Autodesk Inventor part; units mm, degrees
ref_plane "YZ Plane" through (0, 0, 0) normal (1, 0, 0) x (0, 1, 0)
ref_plane "XZ Plane" through (0, 0, 0) normal (0, 1, 0) x (-1, 0, 0)
ref_plane "XY Plane" through (0, 0, 0) normal (0, 0, 1) x (1, 0, 0)
sketch "Esboço1" plane through (0, 0, 0) normal (0, 1, 0) x (-1, 0, 0)
  line L0 (0, 0) -> (22, 0)
  line L1 (22, 0) -> (22, -23.4641)
  line L2 (22, -24) -> (25.6764, -24) construction
  line L3 (0, 0) -> (0, -23.4641)
  line L4 (1.9, -27.8268) -> (1.9, -102.1732)
  line L5 (0, -106.5359) -> (0, -130)
  line L6 (0, -130) -> (22, -130)
  line L7 (22, -130) -> (22, -106.5359)
  line L8 (20.1, -102.1732) -> (20.1, -27.8268)
  line L9 (21.7321, -24.4641) -> (20.3679, -26.8268)
  line L10 (1.6321, -26.8268) -> (0.2679, -24.4641)
  line L11 (20.3679, -103.1732) -> (21.7321, -105.5359)
  line L12 (0.2679, -105.5359) -> (1.6321, -103.1732)
  arc A0 (21.7321, -24.4641) -> (22, -23.4641) centre (20, -23.4641) ccw
  arc A1 (20.3679, -26.8268) -> (20.1, -27.8268) centre (22.1, -27.8268) ccw
  arc A2 (1.9, -27.8268) -> (1.6321, -26.8268) centre (-0.1, -27.8268) ccw
  arc A3 (0, -23.4641) -> (0.2679, -24.4641) centre (2, -23.4641) ccw
  arc A4 (22, -106.5359) -> (21.7321, -105.5359) centre (20, -106.5359) ccw
  arc A5 (20.1, -102.1732) -> (20.3679, -103.1732) centre (22.1, -102.1732) ccw
  arc A6 (1.6321, -103.1732) -> (1.9, -102.1732) centre (-0.1, -102.1732) ccw
  arc A7 (0.2679, -105.5359) -> (0, -106.5359) centre (2, -106.5359) ccw
  line L13 (7.5, -52.4035) -> (7.5, -77.5965)
  spline S0 degree 3 poles (7.5, -52.4035) (7.1712, -52.2005) (6.8736, -51.9509) (6.3593, -51.374) (6.1453, -51.0498) (5.8168, -50.3503) (5.704, -49.9786) (5.5886, -49.2144) (5.5866, -48.826) (5.6404, -48.4433) knots -0.463747 -0.463747 -0.463747 -0.463747 -0.347807 -0.347807 -0.231874 -0.231874 -0.115941 -0.115941 -0.000001 -0.000001 -0.000001 -0.000001
  line L14 (5.6404, -48.4433) -> (6.2661, -43.9914)
  spline S1 degree 3 poles (6.2661, -43.9914) (6.3326, -43.5177) (6.4837, -43.0598) (6.9401, -42.2191) (7.2419, -41.8431) (7.9639, -41.2155) (8.3783, -40.9689) (9.2743, -40.6339) (9.7488, -40.5481) (10.2271, -40.5481) knots -0.574004 -0.574004 -0.574004 -0.574004 -0.430503 -0.430503 -0.287003 -0.287003 -0.143502 -0.143502 -0.000001 -0.000001 -0.000001 -0.000001
  line L15 (10.2271, -40.5481) -> (11.7729, -40.5481)
  spline S2 degree 3 poles (11.7729, -40.5481) (12.2512, -40.5481) (12.7257, -40.6339) (13.6217, -40.9689) (14.0361, -41.2155) (14.7581, -41.8431) (15.0599, -42.2191) (15.5163, -43.0598) (15.6674, -43.5177) (15.7339, -43.9914) knots -0.574004 -0.574004 -0.574004 -0.574004 -0.430503 -0.430503 -0.287003 -0.287003 -0.143502 -0.143502 -0.000001 -0.000001 -0.000001 -0.000001
  line L16 (15.7339, -43.9914) -> (16.3596, -48.4433)
  spline S3 degree 3 poles (16.3596, -48.4433) (16.4134, -48.826) (16.4114, -49.2144) (16.296, -49.9786) (16.1832, -50.3503) (15.8547, -51.0498) (15.6407, -51.374) (15.1264, -51.9509) (14.8288, -52.2005) (14.5, -52.4035) knots -0.463747 -0.463747 -0.463747 -0.463747 -0.347807 -0.347807 -0.231874 -0.231874 -0.115941 -0.115941 -0.000001 -0.000001 -0.000001 -0.000001
  line L17 (14.5, -77.5965) -> (14.5, -52.4035)
  spline S4 degree 3 poles (14.5, -77.5965) (14.8288, -77.7995) (15.1264, -78.0491) (15.6407, -78.626) (15.8547, -78.9502) (16.1832, -79.6497) (16.296, -80.0214) (16.4114, -80.7856) (16.4134, -81.174) (16.3596, -81.5567) knots -0.463747 -0.463747 -0.463747 -0.463747 -0.347807 -0.347807 -0.231874 -0.231874 -0.115941 -0.115941 -0.000001 -0.000001 -0.000001 -0.000001
  line L18 (15.7339, -86.0086) -> (16.3596, -81.5567)
  spline S5 degree 3 poles (15.7339, -86.0086) (15.6674, -86.4823) (15.5163, -86.9402) (15.0599, -87.7809) (14.7581, -88.1569) (14.0361, -88.7845) (13.6217, -89.0311) (12.7257, -89.3661) (12.2512, -89.4519) (11.7729, -89.4519) knots -0.574004 -0.574004 -0.574004 -0.574004 -0.430503 -0.430503 -0.287003 -0.287003 -0.143502 -0.143502 -0.000001 -0.000001 -0.000001 -0.000001
  spline S6 degree 3 poles (10.2271, -89.4519) (9.7488, -89.4519) (9.2743, -89.3661) (8.3783, -89.0311) (7.9639, -88.7845) (7.2419, -88.1569) (6.9401, -87.7809) (6.4837, -86.9402) (6.3326, -86.4823) (6.2661, -86.0086) knots -0.574004 -0.574004 -0.574004 -0.574004 -0.430503 -0.430503 -0.287003 -0.287003 -0.143502 -0.143502 -0.000001 -0.000001 -0.000001 -0.000001
  line L19 (10.2271, -89.4519) -> (11.7729, -89.4519)
  line L20 (5.6404, -81.5567) -> (6.2661, -86.0086)
  spline S7 degree 3 poles (5.6404, -81.5567) (5.5866, -81.174) (5.5886, -80.7856) (5.704, -80.0214) (5.8168, -79.6497) (6.1453, -78.9502) (6.3593, -78.626) (6.8736, -78.0491) (7.1712, -77.7995) (7.5, -77.5965) knots -0.463747 -0.463747 -0.463747 -0.463747 -0.347807 -0.347807 -0.231874 -0.231874 -0.115941 -0.115941 -0.000001 -0.000001 -0.000001 -0.000001
  point P0 (20.1, -27.2909)
  point P1 (0, -24)
  point P2 (1.9, -27.2909)
  point P3 (0, -106)
  point P4 (22, -106)
  point P5 (20.1, -102.7091)
  point P6 (11, -130)
  point P7 (11, -89.4519)
  point P8 (11, -40.5481)
  point P9 (20.1, -65)
  point P10 (14.5, -65)
  dimension "d0" = 22
  dimension "d1" = 24
  dimension "d4" = 3.8
  dimension "d6" = 3.8
  dimension "d7" = 24
  dimension "d8" = 18.2
  dimension "d10" = 0
  dimension "d11" = 130
  dimension "d12" = 1.9
  dimension "d13" = 2
  dimension "d14" = 2
  dimension "d38" = 7
  dimension "d39" = 7
  dimension "d40" = 4.4957
  dimension "d41" = 4.4957
  dimension "d42" = 4.4519
  dimension "d43" = 0.6257
  dimension "d44" = 172
  dimension "d45" = 1.5457
  dimension "d46" = 1.5457
  dimension "d47" = 0.6257
  dimension "d48" = 4.4519
  dimension "d49" = 3.9611
  dimension "d50" = 3.4433
  dimension "d51" = 9.4679
  dimension "d52" = 3.9611
  dimension "d53" = 3.9602
  dimension "d54" = 1.8596
  dimension "d55" = 4.4519
  dimension "d56" = 3.9602
  dimension "d57" = 3.9602
  dimension "d58" = 4.3751
  dimension "d59" = 1.8596
  dimension "d60" = 3.9611
  dimension "d61" = 3.9611
  dimension "d62" = 3.4433
  dimension "d63" = 3.4433
  dimension "d64" = 0
  dimension "d65" = 48.9038
  dimension "d67" = 0
extrude "Extrusão1" add sketch "Esboço1" along normal blind 25.4
sketch "Esboço2" plane through (0, 0, 0) normal (1, 0, 0) x (0, 0, -1)
  line L0 (0, 0) -> (0, 25.4)
  line L1 (0, 25.4) -> (23.4641, 25.4)
  line L2 (130, 0) -> (130, 25.4)
  line L3 (106.5359, 25.4) -> (130, 25.4)
  point P0 (12, 20.2)
  point P1 (12, 5.2)
  point P2 (118, 20.2)
  point P3 (118, 5.2)
  point P4 (11.7321, 25.4)
  dimension "d70" = 15
  dimension "d72" = 25.4
  dimension "d73" = 5.2
  dimension "d74" = 0
  dimension "d75" = 12
  dimension "d76" = 15
  dimension "d77" = 12
  dimension "d78" = 0
  dimension "d79" = 5.2
hole "Furo1" at (0, 20.2, -12) at (0, 5.2, -12) at (0, 20.2, -118) at (0, 5.2, -118) direction (-1, 0, 0) diameter 5 end through all
equation "\"d85\" = Espessura"
equation "\"Raio_vergadura\" = Espessura"
equation "\"Largura_alívio_de_vergadura\" = Espessura"
equation "\"Profundidade_alívio_de_vergadura\" = 0.5 * Espessura"
equation "\"Tamanho_alívio_de_dobra\" = 4 * Espessura"
equation "\"Remanescente_mínimo\" = 2 * Espessura"
equation "\"Raiodetransição\" = Raio_vergadura"
equation "\"Tamanho_de_raio_de_Jacobi\" = Raio_vergadura"
equation "\"TamanhoFolga\" = Espessura"
properties part number "Célula de carga" material "Alumínio 6061"
Could you check a few things on this model? Use its own coordinates, in mm. A direction names the side the tool comes from. Round coordinates to 2 decimals unless told otherwise and drop trailing zeros. Loops run counter-clockwise (first coordinate to the right, second up) from the corner with the lowest first, then second, coordinate; pieces in that order, holes last. Notation, with made-up numbers: (54.5, -20.75) -> (107.5, -20.75) arc R32 ccw to (107.5, 16.25) -> close; hole circle Ø2 at (46.5, 87.25). An arc over 180 degrees is marked (long way). One line per question, with ' | ' between items.
(1) For pin 1 Ø8 at (x, z) = (-8.5, -73) entering from -Y; pin 2 Ø3 at (y, z) = (20.5, -86) entering from +X; pin 3 Ø12 at (y, z) = (10.5, -81) entering from -X, each with a flat end and sliding along its axis, tell me the tip position at first contact or that it passes through.
Model answer:
pin 1: stops at y = 0 | pin 2: stops at x = -1.9 | pin 3: stops at x = -20.1
(2) If we section it at D-D on x = -18.75: List the corners of the cut face in (y, z) for me.
Model answer:
outline: (0, -130) -> (25.4, -130) -> (25.4, 0) -> (0, 0) -> close; hole circle Ø5 at (5.2, -118); hole circle Ø5 at (5.2, -12); hole circle Ø5 at (20.2, -118); hole circle Ø5 at (20.2, -12)
(3) If I drill on probe 1 along Y at (x, z) = (-5, -12); probe 2 along Z at (x, y) = (-13, 20.2); probe 3 along Z at (x, y) = (-6.75, 20.2), over which ranges is the centre line in solid material (lowest first)?
Model answer:
probe 1: y = 0 to 2.7, 7.7 to 17.7, 22.7 to 25.4 | probe 2: z = -130 to -120.5, -115.5 to -89.26, -40.74 to -14.5, -9.5 to 0 | probe 3: z = -130 to -120.5, -115.5 to -87.43, -78.19 to -51.81, -42.57 to -14.5, -9.5 to 0
(4) For faces 1 (the face through (-7.5, 13, -65)), 2 (the face through (-21.04, 12.52, -104.34)), 3 (the face through (-16, 25.4, -64)), which set-ups out of +Z, -Z, +X, -X, +Y, -Y let a thin tool reach every point of the face, with its end or its side?
Model answer:
face 1: +Y, -Y | face 2: -X, +Y, -Y | face 3: +Z, -Z, +X, -X, +Y
(5) Thinking about a two-plate mould opening in X: for faces 4 (the face through (-0.96, 12.52, -25.66)), 5 (the face through (-5.95, 12.52, -83.75)), 6 (the face through (-22, 13, -12)), which applies, released by +X, released by -X, zero draft, split by the parting line, or undercut?
Model answer:
face 4: released by +X | face 5: undercut | face 6: released by -X
(6) If we section it at C-C on z = -12: List the corners of the cut face in (x, y) for me, and give its area (3 significant figures).
Model answer:
outline: (-22, 0) -> (0, 0) -> (0, 2.7) -> (-22, 2.7) -> close; (-22, 7.7) -> (0, 7.7) -> (0, 17.7) -> (-22, 17.7) -> close; (-22, 22.7) -> (0, 22.7) -> (0, 25.4) -> (-22, 25.4) -> close | area: 339 mm^2
(7) If we section it at A-A on z = -53.5: List the corners of the cut face in (x, y) for me.
Model answer:
outline: (-20.1, 0) -> (-14.5, 0) -> (-14.5, 25.4) -> (-20.1, 25.4) -> close; (-7.5, 0) -> (-1.9, 0) -> (-1.9, 25.4) -> (-7.5, 25.4) -> close
(8) If we section it at B-B on y = 5.2: Count the separate pieces of the cut face and the enclosed holes in it, and give its area (3 significant figures).
Model answer:
separate pieces: 3 | enclosed holes: 1 | area: 1,940 mm^2
